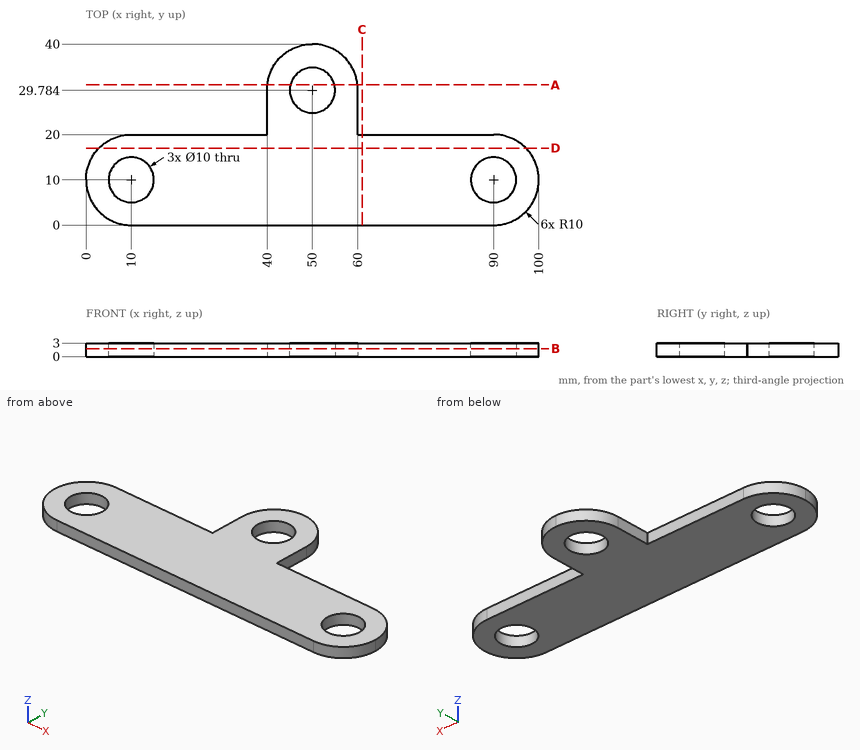
Answer from the drawing. Dimensions are ordinates in mm from the lowest x, y and z of the part. Round coordinates to 2 decimals unless told otherwise and drop trailing zeros. Write each loop counter-clockwise with the first axis right and the second up, starting at its lowest first coordinate (ties: lowest second). Pieces come first, ordered by that corner, then holes. Notation, with made-up numbers: (12.25, -4) -> (68.25, -4) arc R27 cw to (68.25, 13) -> close; hole circle Ø8 at (30, 49.25). An arc over 180 degrees is marked (long way). Answer in a Markdown table with one row per item. Add a question column.
1) Consider line 1 (Y direction, x = 90, z = 2.1); line 2 (X direction, y = 8.5, z = 1.65); line 3 (X direction, y = 30, z = 2.1) (1 decimal). Determine where each line is inside the solid, lowest interval first.
2) Find section D-D, the plane y = 17. Determine the outline of the cut face in (x, z).
3) Given P1, Ø8, axis at x = 50, y = 29.78, coming from the +Z side; P2, Ø1.5, axis at y = 5.5, z = 0.5, coming from the -X side; P3, Ø1.5, axis at y = 12, z = 2, coming from the -X side; P4, Ø1, axis at y = 17.5, z = 0.5, coming from the +X side, each flat-ended and moving along its own axis, determine where each tip first touches the part or whether it passes through.
4) Find section B-B, the plane z = 1.8. State how many separate pieces and enclosed holes the cut face has, and give its area (3 significant figures).
5) Find section C-C, the plane x = 61. Determine the outline of the cut face in (y, z).
6) Find section A-A, the plane y = 31. Determine the outline of the cut face in (x, z).
Findings below:
| question | item | result |
|---|---|---|
| 1 | line 1 | 0 to 5, 15 to 20 |
| 1 | line 2 | 0.11 to 5.23, 14.77 to 85.23, 94.77 to 99.89 |
| 1 | line 3 | 40 to 45, 55 to 60 |
| 2 | outline | (2.86, 0) -> (97.14, 0) -> (97.14, 3) -> (2.86, 3) -> close |
| 3 | P1 | through |
| 3 | P2 | x = 0.73 |
| 3 | P3 | x = 0.08 |
| 3 | P4 | x = 97.14 |
| 4 | separate pieces | 1 |
| 4 | enclosed holes | 3 |
| 4 | area | 2,040 mm² |
| 5 | outline | (0, 0) -> (20, 0) -> (20, 3) -> (0, 3) -> close |
| 6 | outline | (40.05, 0) -> (45.15, 0) -> (45.15, 3) -> (40.05, 3) -> close; (54.85, 0) -> (59.95, 0) -> (59.95, 3) -> (54.85, 3) -> close |
